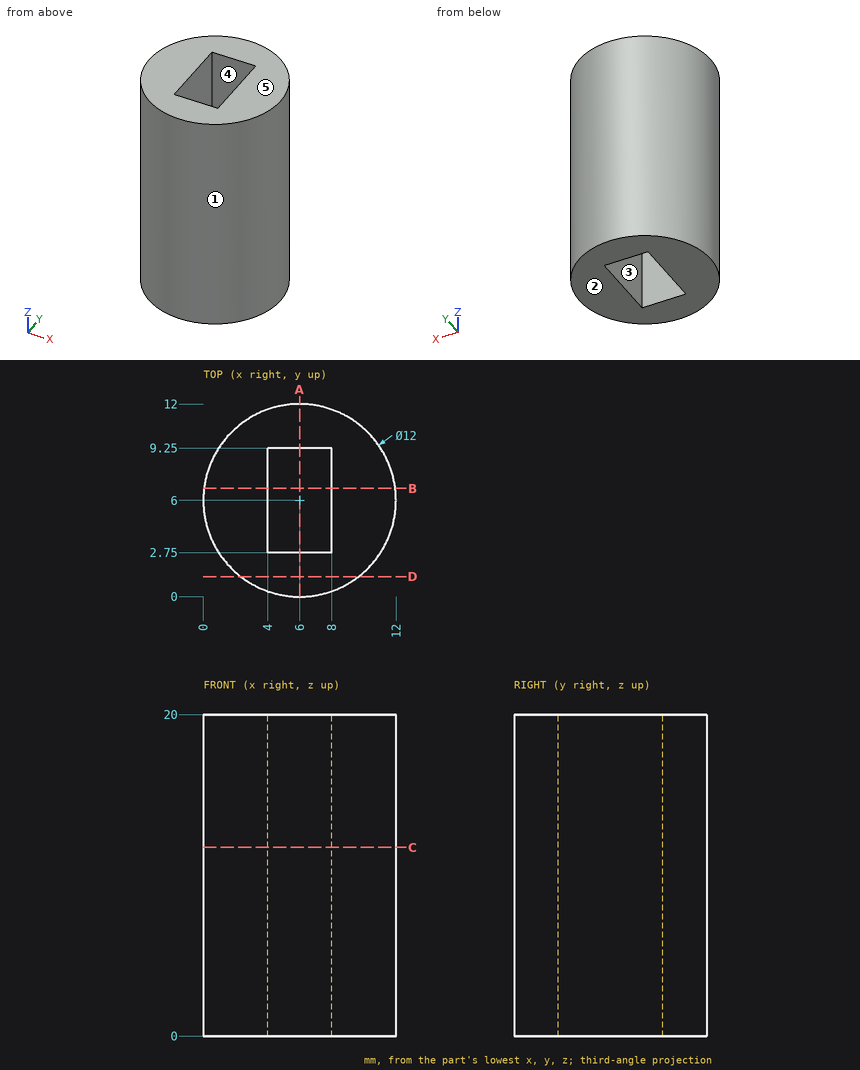
The drawing under review shows one solid part. Ordinate dimensions are in mm from its lowest x, y, z. A direction names the side the tool comes from. Round coordinates to 2 decimals unless told otherwise and drop trailing zeros. Loops run counter-clockwise (first coordinate to the right, second up) from the corner with the lowest first, then second, coordinate; pieces in that order, holes last. Notation, with made-up numbers: M 63.25,23 L 75.25,23 A13 ccw 75.25,45 Z; hole C 25,-2 d10. An arc over 180 degrees is marked long. Answer as CSV lines item,"result". Start each with the question number.
Item 1: Insertion check: P1, Ø1, axis at x = 5.5, y = 1.5, coming from the -Z side; P2, Ø2, axis at y = 10.5, z = 11, coming from the -X side. Each pin has a flat end and moves straight along its axis. Give the tip position at first contact, or say it passes through.
Item 2: For the marked faces 4 and 5, list the 3-axis set-ups (+Z, -Z, +X, -X, +Y, -Y) from which the entire face can be reached by the end or side of a thin tool; tool diameter is ignored.
Item 3: Mouldability with a two-part tool opening along Y and no side actions: class the marked faces 1, 2 and 3 as released by +Y, released by -Y, zero draft, split by the parting line, or undercut.
Item 4: Consider section A-A (x = 6). Write out the cut boundary in (y, z).
Item 5: Consider section D-D (y = 1.25). Write out the cut boundary in (x, z), then the cut area to 3 significant figures.
Item 6: Wall thickness on line 1 (Y direction, x = 5.5, z = 19.25); line 2 (Y direction, x = 7.75, z = 17); line 3 (X direction, y = 5, z = 11.5): over which ranges is each line inside the solid? List them lowest first. Write a range as [from, to].
Item 7: Consider section C-C (z = 11.75). Write out the cut boundary in (x, y), then the cut area to 3 significant figures.
Item 8: Consider section B-B (y = 6.75). Write out the cut boundary in (x, z).
Answer:
1,P1,"stops at z = 0"
1,P2,"stops at x = 1.13"
2,face 4,"+Z, -Z"
2,face 5,"+Z, +X, -X, +Y, -Y"
3,face 1,"split by the parting line"
3,face 2,"zero draft"
3,face 3,"undercut"
4,outline,"M 0,0 L 2.75,0 L 2.75,20 L 0,20 Z; M 9.25,0 L 12,0 L 12,20 L 9.25,20 Z"
5,outline,"M 2.33,0 L 9.67,0 L 9.67,20 L 2.33,20 Z"
5,area,"147 mm^2"
6,line 1,"y = [0.02, 2.75], [9.25, 11.98]"
6,line 2,"y = [0.26, 2.75], [9.25, 11.74]"
6,line 3,"x = [0.08, 4], [8, 11.92]"
7,outline,"C 6,6 d12; hole M 4,2.75 L 8,2.75 L 8,9.25 L 4,9.25 Z"
7,area,"87.1 mm^2"
8,outline,"M 0.05,0 L 4,0 L 4,20 L 0.05,20 Z; M 8,0 L 11.95,0 L 11.95,20 L 8,20 Z"
